```python
from build123d import *

# Parameters (mm, degrees)
F0_W     = 203.2
F0_H     = 101.6
F1_DEPTH = 101.6
F2_W     = 152.4
F2_H     = 76.2
F3_DEPTH = 76.2
F5_DEPTH = 152.4


with BuildPart() as f1:
    # F0 (on Top) → F1 (new body)
    with BuildSketch(Plane.XY):
        Rectangle(F0_W, F0_H)
    extrude(amount=F1_DEPTH)

    # F2 (on face) → F3 (cut)
    with BuildSketch(Plane.XY.offset(101.6)):
        with Locations((0, -12.7)):
            Rectangle(F2_W, F2_H)
    extrude(amount=-F3_DEPTH, mode=Mode.SUBTRACT)

    # F4 (on face) → F5 (join)
    with BuildSketch(Plane.YZ.offset(-76.2)):
        Polygon((25.4, 25.4), (25.4, 101.6), (-50.8, 25.4), align=None)
    extrude(amount=F5_DEPTH)


solid = f1.part
```
CAD build for the part. Positions are in the model's coordinates, mm. A direction names the side the tool comes from. Coordinates: 2 decimals unless noted, no trailing zeros. Order: outer loops, then holes, each group sorted by start corner. A loop starts at its lowest first (then second) coordinate and runs counter-clockwise, first axis right, second up. Notation, with made-up numbers: (-16.5, -2.5) - (-7.5, -2.5) arc R17 cw to (-7.5, 17.5) - close; hole circle Ø9 at (0, 43.25). An arc over 180 degrees is marked (long way). Use a Markdown table: item, result. Add a question column.
(1) Drill centre lines: line 1 along X through (y, z) = (-36.5, 50); line 2 along Y through (x, z) = (27, 75); line 3 along Z through (x, y) = (24, -29). Where is each one in solid material? Low to high. Write a range as [from, to].
(2) Pull direction X, two halves, no side cores. Call faces 1 (the face through (-1, 35, 101.6)), 2 (the face through (-76.2, -22, 73)), 3 (the face through (-101.6, -1, 50)): +X half, -X half, draft (parallel to the pull), parting line (faces both ways), or undercut.
(3) Saw through at B-B (z = 36). Give the cut face in (x, y).
(4) Flat gauge pins, fed straight in: pin 1 (2 mm diameter, centred on x = 57.5, y = 24, fed in from +Z); pin 2 (4 mm diameter, centred on x = 43.5, y = 15.5, fed in from +Z); pin 3 (3 mm diameter, centred on x = 51.5, y = 23, fed in from +Z). Where does each tip first touch, or does it go through?
(5) Saw through at A-A (y = -32). Give the cut face in (x, z).
(6) Saw through at C-C (x = -4). Give the cut face in (y, z).
(7) Which spindle directions (+Z, -Z, +X, -X, +Y, -Y) get a long thin tool onto all of the face, cutting with end or side? Do faces 4 (the face through (-1, 50.8, 50)), 5 (the face through (-1.1, -12.2, 64)). Say none if no direction does.
Solved:
| question | item | result |
|---|---|---|
| 1 | line 1 | x = [-101.6, -76.2], [76.2, 101.6] |
| 1 | line 2 | y = [-1.2, 50.8] |
| 1 | line 3 | z = [0, 47.2] |
| 2 | face 1 | draft |
| 2 | face 2 | undercut |
| 2 | face 3 | -X half |
| 3 | outline | (-101.6, -50.8) - (-76.2, -50.8) - (-76.2, -40.2) - (76.2, -40.2) - (76.2, -50.8) - (101.6, -50.8) - (101.6, 50.8) - (-101.6, 50.8) - close |
| 4 | pin 1 | stops at z = 101.2 |
| 4 | pin 2 | stops at z = 93.7 |
| 4 | pin 3 | stops at z = 100.7 |
| 5 | outline | (-101.6, 0) - (101.6, 0) - (101.6, 101.6) - (76.2, 101.6) - (76.2, 44.2) - (-76.2, 44.2) - (-76.2, 101.6) - (-101.6, 101.6) - close |
| 6 | outline | (-50.8, 0) - (50.8, 0) - (50.8, 101.6) - (25.4, 101.6) - (-50.8, 25.4) - close |
| 7 | face 4 | +Z, -Z, +X, -X, +Y |
| 7 | face 5 | +Z, -Y |
